Geometry check sheet. Reference: drawing and pictorial views, mm from the part's lowest x, y, z. A direction names the side the tool comes from. Round coordinates to 2 decimals unless told otherwise and drop trailing zeros. Write each loop counter-clockwise with the first axis right and the second up, starting at its lowest first coordinate (ties: lowest second). Pieces come first, ordered by that corner, then holes. Notation, with made-up numbers: M -22.5,3.25 L 23.5,3.25 A31 ccw 23.5,38.25 Z; hole C 46.25,-22.75 d4. An arc over 180 degrees is marked long. Use a Markdown table: item, result. Add a question column.
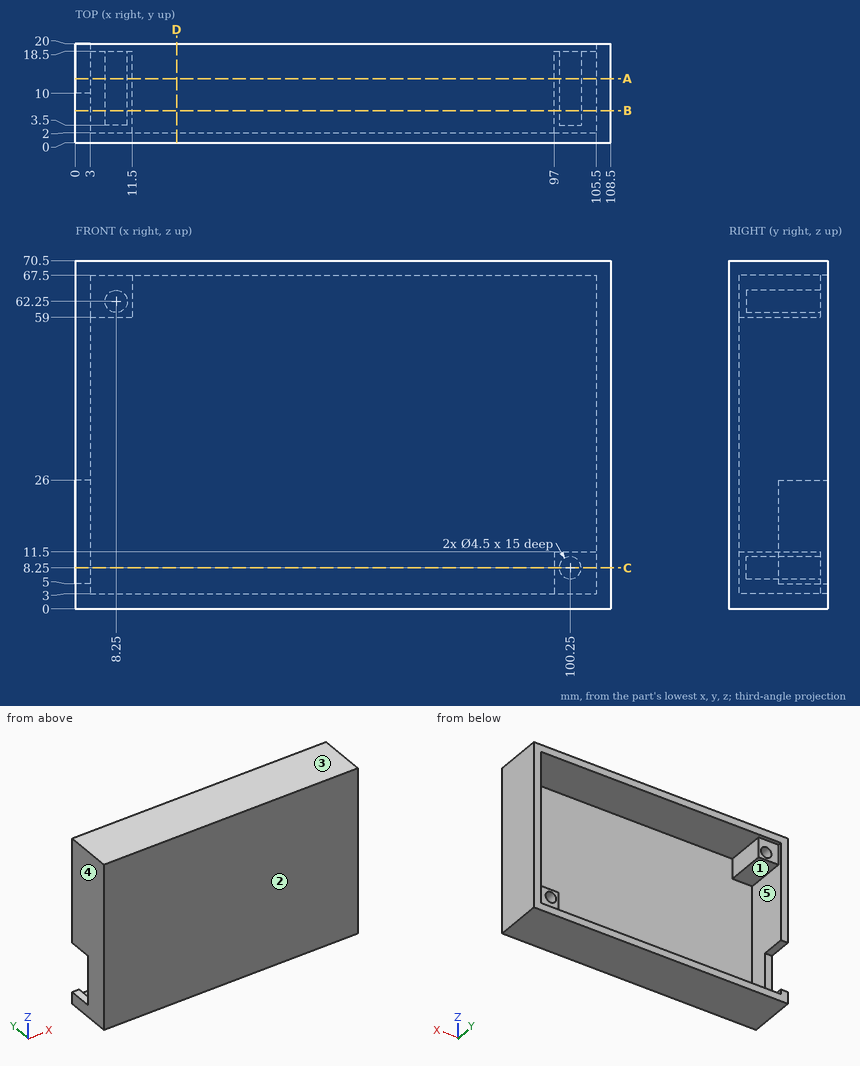
1. Cross-section at C-C on z = 8.25. Enter the section's corners in (x, y), plus the area to 3 significant figures.
2. Scan lines: line 1 along X through (y, z) = (11, 62.25); line 2 along Z through (x, y) = (100.25, 15.25); line 3 along X through (y, z) = (9.5, 8.25). Record each from-to range of solid material in increasing order. Write a range as from..to.
3. Cross-section at D-D on x = 20.5. Enter the section's corners in (y, z).
4. Cross-section at A-A on y = 13. Enter the section's corners in (x, z), plus the area to 3 significant figures.
5. Cross-section at B-B on y = 6.5. Enter the section's corners in (x, z).
6. Depth check by flat-ended pin: pin 1 Ø1 at (x, z) = (85.5, 26.5) entering from +Y; pin 2 Ø0.9 at (x, z) = (1.5, 17.5) entering from +Y; pin 3 Ø3.5 at (x, z) = (7, 61.5) entering from +Y. Enter the tip coordinate at first touch or a pass-through.
7. Release check for a two-part mould opening along Z. For the marked faces 1, 2 and 3 record: +Z half, -Z half, draft (parallel to the pull), parting line (faces both ways), or undercut.
8. Access from +Z, -Z, +X, -X, +Y, -Y to the whole of each face (thin tool, end or side, straight path). Record for the marked faces 4 and 5.
Answer:
| question | item | result |
|---|---|---|
| 1 | outline | M 0,0 L 108.5,0 L 108.5,20 L 105.5,20 L 105.5,18.5 L 102.5,18.5 L 102.5,3.5 L 98,3.5 L 98,18.5 L 97,18.5 L 97,2 L 3,2 L 3,10 L 0,10 Z |
| 1 | area | 368 mm^2 |
| 2 | line 1 | x = 0..6, 10.5..11.5, 105.5..108.5 |
| 2 | line 2 | z = 0..6, 10.5..11.5, 67.5..70.5 |
| 2 | line 3 | x = 0..3, 97..98, 102.5..108.5 |
| 3 | outline | M 0,0 L 20,0 L 20,3 L 2,3 L 2,67.5 L 20,67.5 L 20,70.5 L 0,70.5 Z |
| 4 | outline | M 0,0 L 108.5,0 L 108.5,70.5 L 0,70.5 L 0,26 L 3,26 L 3,59 L 11.5,59 L 11.5,67.5 L 105.5,67.5 L 105.5,11.5 L 97,11.5 L 97,3 L 3,3 L 3,5 L 0,5 Z; hole C 8.25,62.25 d4.5; hole C 100.25,8.25 d4.5 |
| 4 | area | 1,090 mm^2 |
| 5 | outline | M 0,0 L 108.5,0 L 108.5,70.5 L 0,70.5 Z; hole M 3,3 L 97,3 L 97,11.5 L 105.5,11.5 L 105.5,67.5 L 11.5,67.5 L 11.5,59 L 3,59 Z; hole C 8.25,62.25 d4.5; hole C 100.25,8.25 d4.5 |
| 6 | pin 1 | stops at y = 2 |
| 6 | pin 2 | stops at y = 10 |
| 6 | pin 3 | stops at y = 18.5 |
| 7 | face 1 | undercut |
| 7 | face 2 | draft |
| 7 | face 3 | +Z half |
| 8 | face 4 | +Z, -Z, -X, +Y, -Y |
| 8 | face 5 | +Y |
